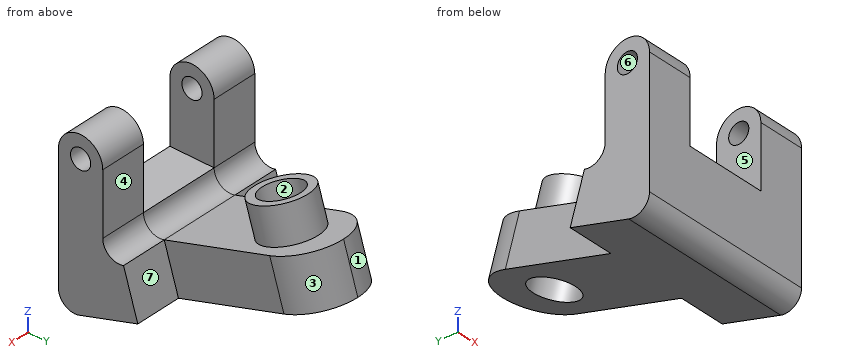
from build123d import *

# Parameters (mm, degrees)
SKETCH1_R                      = 1.5875
BOSS_EXTRUDE1_DEPTH            = 27.305
FILLET1_R                      = 2.54
CUT_EXTRUDE1_REACH             = 49.512
SKETCH2_W                      = 12.7
SKETCH2_H                      = 10.26762413
CUT_EXTRUDE1_DIRECTION_2_DEPTH = 48.511945714
SKETCH3_R                      = 4.445
SKETCH3_R_2                    = 3.175
BOSS_EXTRUDE2_DEPTH            = 5.43375
SKETCH4_R                      = 3.4925
CUT_EXTRUDE2_DEPTH             = 7.673839963
CUT_EXTRUDE3_DEPTH             = 7.3025
CUT_EXTRUDE4_DEPTH             = 7.3025
BOSS_EXTRUDE3_DEPTH            = 12.7
FILLET2_R                      = 6.35


with BuildPart() as part:
    # Sketch1 → Boss-Extrude1 (new body)
    with BuildSketch(Plane(origin=(0, 0, 0), x_dir=(0, 0, -1), z_dir=(1, 0, 0))):
        with BuildLine():
            Line((0, 3.4925), (13.208, 3.4925))
            Line((13.208, 3.4925), (5.261420462, 29.48459049))
            Line((5.261420462, 29.48459049), (12.599950115, 31.728204162))
            Line((12.599950115, 31.728204162), (23.368, -3.4925))
            Line((23.368, -3.4925), (0, -3.4925))
            ThreePointArc((0, -3.4925), (-3.4925, 0), (0, 3.4925))
        make_face()
        Circle(SKETCH1_R, mode=Mode.SUBTRACT)
    extrude(amount=BOSS_EXTRUDE1_DEPTH)

    # Fillet1
    fillet1_edges = [part.edges().sort_by_distance(p)[0] for p in [
        (13.6525, 3.4925, -13.208),
        (13.6525, -3.4925, -23.368),
    ]]
    fillet(fillet1_edges, radius=FILLET1_R)

    # Cut-Extrude1: up to this plane
    cut_extrude1_end = Plane(origin=(27.305, 3.4925, -13.208), z_dir=(0, 0.292371704722731, -0.9563047559630373))
    # Sketch2 → Cut-Extrude1 (cut, up to the surface)
    with BuildSketch(Plane.XY, mode=Mode.PRIVATE) as cut_extrude1_sk1:
        with Locations((13.6525, 1.641312065)):
            Rectangle(SKETCH2_W, SKETCH2_H)
    cut_extrude1_tool1 = split(extrude(cut_extrude1_sk1.sketch, amount=-CUT_EXTRUDE1_REACH, mode=Mode.PRIVATE), bisect_by=cut_extrude1_end, keep=Keep.BOTH, mode=Mode.PRIVATE)
    add(cut_extrude1_tool1.solids().sort_by_distance((13.6525, 1.641312, 0))[0], mode=Mode.SUBTRACT)

    # Sketch2 → Cut-Extrude1 direction 2 (cut)
    with BuildSketch(Plane.XY):
        with Locations((13.6525, 1.641312065)):
            Rectangle(SKETCH2_W, SKETCH2_H)
    extrude(amount=CUT_EXTRUDE1_DIRECTION_2_DEPTH, mode=Mode.SUBTRACT)

    # Sketch3 → Boss-Extrude2 (add)
    with BuildSketch(Plane(origin=(0, 3.991453073, -13.055454737), x_dir=(1, 0, 0), z_dir=(0, -0.2923717047227311, 0.9563047559630372))):
        with Locations(Location((13.6525, 18.054125632, 0), (0, 0, 90))):
            Circle(SKETCH3_R)
        with Locations(Location((13.6525, 18.054125632, 0), (0, 0, 270))):
            Circle(SKETCH3_R_2, mode=Mode.SUBTRACT)
    extrude(amount=BOSS_EXTRUDE2_DEPTH)

    # Sketch4 → Cut-Extrude2 (cut)
    with BuildSketch(Plane(origin=(0, 3.991453073, -13.055454737), x_dir=(1, 0, 0), z_dir=(0, -0.29237170472273094, 0.9563047559630372))):
        with Locations(Location((13.6525, 18.054125632, 0), (0, 0, 270))):
            Circle(SKETCH4_R)
    extrude(amount=-CUT_EXTRUDE2_DEPTH, mode=Mode.SUBTRACT)

    # Sketch5 → Cut-Extrude3 (cut)
    with BuildSketch(Plane.ZY):
        Polygon((-12.599950115, 31.728204162), (-5.261420462, 29.48459049), (-12.204401088, 6.77512413), (-19.542930741, 9.018737802), align=None)
    extrude(amount=-CUT_EXTRUDE3_DEPTH, mode=Mode.SUBTRACT)

    # Sketch6 → Cut-Extrude4 (cut)
    with BuildSketch(Plane(origin=(27.305, 0, 0), x_dir=(0, 0, -1), z_dir=(1, 0, 0))):
        Polygon((12.599950115, 31.728204162), (5.261420462, 29.48459049), (12.204401088, 6.77512413), (19.542930741, 9.018737802), align=None)
    extrude(amount=-CUT_EXTRUDE4_DEPTH, mode=Mode.SUBTRACT)

    # Sketch7 → Boss-Extrude3 (add)
    with BuildSketch(Plane.ZY.offset(-20.0025)):
        with BuildLine():
            Line((-9.775387008, 3.4925), (-9.775387008, -3.4925))
            Line((-9.775387008, -3.4925), (-15.34352881, -3.4925))
            Line((-15.34352881, -3.4925), (-12.204401088, 6.77512413))
            ThreePointArc((-12.204401088, 6.77512413), (-11.817183434, 4.521650122), (-9.775387008, 3.4925))
        make_face()
    extrude(amount=BOSS_EXTRUDE3_DEPTH)

    # Fillet2
    fillet2_edges = [part.edges().sort_by_distance(p)[0] for p in [
        (20.0025, 30.606397326, -8.930685288),
        (7.3025, 30.606397326, -8.930685288),
    ]]
    fillet(fillet2_edges, radius=FILLET2_R - 0.0001)  # a hair under: the kernel refuses the full size


solid = part.part
Source: CAD feature listing. Evaluate the final solid. Frame: model axes, mm. Face numbers are marked on the shaded views. A direction names the side the tool comes from. Coordinates: 2 decimals unless noted, no trailing zeros. Loops run counter-clockwise (first coordinate to the right, second up) from the corner with the lowest first, then second, coordinate; pieces in that order, holes last. Notation, with made-up numbers: M 50.25,12.25 L 93.25,12.25 A20 ccw 93.25,27.25 Z; hole C -13.5,12.5 d4. An arc over 180 degrees is marked long. Answer in a Markdown table with one row per item.
Q1. Section C-C on z = -6. State how many separate pieces and enclosed holes the cut face has, plus the area to 3 significant figures.
Answers below:
| item | result |
|---|---|
| separate pieces | 4 |
| enclosed holes | 1 |
| area | 153 mm^2 |
Q2. Section B-B on y = 1. Return the cut outline in (x, z) (1 decimal).
Answers below:
| item | result |
|---|---|
| outline | M 0,-22 L 27.3,-22 L 27.3,-1.2 L 20,-1.2 L 20,-9.8 L 7.3,-9.8 L 7.3,-1.2 L 0,-1.2 Z; M 0,1.2 L 7.3,1.2 L 7.3,3.3 L 0,3.3 Z; M 20,1.2 L 27.3,1.2 L 27.3,3.3 L 20,3.3 Z |
Q3. Draft query along X for the marked faces 1, 2 and 3. Return one class per face: pulls with the +X half, pulls with the -X half, needs draft (parallel to the pull), parting line crosses it, or undercut.
Answers below:
| item | result |
|---|---|
| face 1 | pulls with the -X half |
| face 2 | undercut |
| face 3 | pulls with the +X half |
Q4. Section D-D on z = -19. Return the cut outline in (x, y) (1 decimal).
Answers below:
| item | result |
|---|---|
| outline | M 0,-3.5 L 27.3,-3.5 L 27.3,8.9 L 20,8.9 L 20,10.8 L 7.3,10.8 L 7.3,8.9 L 0,8.9 Z |
Q5. Set-up query: the marked faces 4, 5, 6 and 7. Return all of +Z, -Z, +X, -X, +Y, -Y with unobstructed straight access to the full face (end or side cutting, diameter ignored); none if empty.
Answers below:
| item | result |
|---|---|
| face 4 | +Z, +X, -X, +Y |
| face 5 | +Z, -Y |
| face 6 | +X, -X |
| face 7 | +Z, +X, +Y |
Q6. Section A-A on x = 6.5. Return the cut outline in (y, z) (1 decimal), plus the area to 3 significant figures.
Answers below:
| item | result |
|---|---|
| outline | M -3.5,-19.9 A2.5 ccw -0.2,-22.4 L 9,-19.5 L 6.8,-12.2 A2.5 cw 3.5,-9.8 L 3.5,0 A3.5 ccw -3.5,0 Z; hole C 0,0 d3.2 |
| area | 202 mm^2 |
Q7. Ray query, probe 1 along X at (y, z) = (-1, -8.5) (1 decimal); probe 2 along Y at (x, z) = (25.5, -6.5); probe 3 along Z at (x, y) = (11.5, -1). Return the intervals inside material, ascending. Write a range as from..to.
Answers below:
| item | result |
|---|---|
| probe 1 | x = 0..7.3, 20..27.3 |
| probe 2 | y = -3.49..3.49 |
| probe 3 | z = -22.47..-9.78 |
Q8. First-contact query: pin 1 (3.5 mm diameter, centred on x = 3.5, z = -4.5, fed in from +Y); pin 2 (1.5 mm diameter, centred on x = 10, z = -7, fed in from -Y); pin 3 (10 mm diameter, centred on y = 22, z = -6, fed in from +X). Flat tips, straight axial feed; report the tip coordinate or a pass-through.
Answers below:
| item | result |
|---|---|
| pin 1 | stops at y = 3.49 |
| pin 2 | stops at y = 17.46 |
| pin 3 | stops at x = 20 |
